Model file for the job. Use its own axes, mm. A direction names the side the tool comes from. Round coordinates to 2 decimals unless told otherwise and drop trailing zeros. Use one line per item in the form item = value.
from build123d import *

# Parameters (mm, degrees)
BOSS_EXTRU_1_DEPTH      = 2
CONG_1_R                = 10
ENL_V_MAT_EXTRU_1_DEPTH = 2
BOSS_EXTRU_2_DEPTH      = 0.6
CONG_2_R                = 10
ESQUISSE3_R             = 1.15
ENL_V_MAT_EXTRU_2_DEPTH = 10
CHANFREIN1_SIZE         = 0.5
CHANFREIN3_SIZE         = 0.6


with BuildPart() as part:
    # Esquisse1 → Boss.-Extru.1 (new body)
    with BuildSketch(Plane.XY):
        Polygon((-40.879571388, 34.615718895), (81.042798068, 34.615718895), (104.193503713, 7.025782272), (38.617977526, -93.674532757), (1.545249154, -93.674532757), (-64.030277033, 7.025782272), align=None)
    extrude(amount=BOSS_EXTRU_1_DEPTH)

    # Congé1
    cong_1_edges = [part.edges().sort_by_distance(p)[0] for p in [
        (-40.879571388, 34.615718895, 1),
        (81.042798068, 34.615718895, 1),
        (104.193503713, 7.025782272, 1),
        (38.617977526, -93.674532757, 1),
        (1.545249154, -93.674532757, 1),
        (-64.030277033, 7.025782272, 1),
    ]]
    fillet(cong_1_edges, radius=CONG_1_R)

    # Esquisse2 → Enlèv. mat.-Extru.1 (cut)
    with BuildSketch(Plane.XY.offset(2)):
        Polygon((-36.216494806, 24.615718895), (-51.607204261, 6.27378561), (6.96667711, -83.674532757), (33.19654957, -83.674532757), (91.770430941, 6.27378561), (76.379721487, 24.615718895), align=None)
    extrude(amount=-ENL_V_MAT_EXTRU_1_DEPTH, mode=Mode.SUBTRACT)

    # Esquisse4 → Boss.-Extru.2 (add)
    with BuildSketch(Plane(origin=(0, 0, 0), x_dir=(-1, 0, 0), z_dir=(0, 0, -1))):
        Polygon((-78.244952119, 28.615718895), (-96.73966005, 6.574584275), (-35.365120753, -87.674532757), (-4.798105928, -87.674532757), (56.57643337, 6.574584275), (38.081725439, 28.615718895), align=None)
        Polygon((-76.379721487, 24.615718895), (-91.770430941, 6.27378561), (-33.19654957, -83.674532757), (-6.96667711, -83.674532757), (51.607204261, 6.27378561), (36.216494806, 24.615718895), align=None, mode=Mode.SUBTRACT)
    extrude(amount=BOSS_EXTRU_2_DEPTH)

    # Congé2
    cong_2_edges = [part.edges().sort_by_distance(p)[0] for p in [
        (-36.216494806, 24.615718895, 0.7),
        (76.379721487, 24.615718895, 0.7),
        (91.770430941, 6.27378561, 0.7),
        (33.19654957, -83.674532757, 0.7),
        (6.96667711, -83.674532757, 0.7),
        (-51.607204261, 6.27378561, 0.7),
    ]]
    fillet(cong_2_edges, radius=CONG_2_R)

    # Esquisse3 → Enlèv. mat.-Extru.2 (cut)
    with BuildSketch(Plane.XY.offset(2)):
        with Locations((20.08161334, -91.058073416)):
            Circle(ESQUISSE3_R)
        with Locations((-28.872824595, -42.931783887)):
            Circle(ESQUISSE3_R)
        with Locations((20.08161334, 32.415718895)):
            Circle(ESQUISSE3_R)
        with Locations((90.076701777, 20.426939275)):
            Circle(ESQUISSE3_R)
        with Locations((69.036051275, -42.931783887)):
            Circle(ESQUISSE3_R)
        with Locations((-49.913475097, 20.426939275)):
            Circle(ESQUISSE3_R)
    extrude(amount=-ENL_V_MAT_EXTRU_2_DEPTH, mode=Mode.SUBTRACT)

    # Chanfrein1
    chanfrein1_edges = [part.edges().sort_by_distance(p)[0] for p in [
        (-51.063475097, 20.426939275, 2),
        (67.886051275, -42.931783887, 2),
        (88.926701777, 20.426939275, 2),
        (18.93161334, 32.415718895, 2),
        (-30.022824595, -42.931783887, 2),
        (18.93161334, -91.058073416, 2),
    ]]
    chamfer(chanfrein1_edges, length=CHANFREIN1_SIZE)

    # Chanfrein3
    chanfrein3_edges = [part.edges().sort_by_distance(p)[0] for p in [
        (87.492306084, 17.595151585, -0.6),
        (20.08161334, 28.615718895, -0.6),
        (-47.329079404, 17.595151585, -0.6),
        (-25.889163721, -40.549974241, -0.6),
        (20.08161334, -87.674532757, -0.6),
        (66.052390401, -40.549974241, -0.6),
    ]]
    chamfer(chanfrein3_edges, length=CHANFREIN3_SIZE - 0.0001)  # a hair under: the kernel refuses the full size


solid = part.part
(1) Pin check, flat tips, straight feed: pin 1 (1.5 mm diameter, centred on x = 78.5, z = 1.5, fed in from +Y); pin 2 (1.8 mm diameter, centred on x = 20.08, y = 32.42, fed in from +Z); pin 3 (3.5 mm diameter, centred on x = -28.87, y = -42.93, fed in from -Z); pin 4 (3 mm diameter, centred on x = 69.04, y = -42.93, fed in from +Z). Stop position of each tip, or through.
Report:
pin_1 = 34.52
pin_2 = through
pin_3 = 0
pin_4 = 1.85
(2) Slice it at B-B on z = 0.45. Count the separate pieces of the cut face and the enclosed holes in it, then the cut area to 3 significant figures.
Report:
separate_pieces = 1
enclosed_holes = 7
area = 4,340 mm2
(3) Pull direction Y, two halves, no side cores. Call faces 1 (the face through (7.56, -82.43, 0.72)), 2 (the face through (57, -48, 2)), 3 (the face through (80.55, 33.704, 1.014)), 4 (the face through (83.14, 16.56, 0.72)): released by +Y, released by -Y, zero draft, split by the parting line, or undercut.
Report:
face_1 = undercut
face_2 = zero draft
face_3 = released by +Y
face_4 = undercut
(4) Probe probe 1 along X at (y, z) = (20.5, 1.8); probe 2 along Y at (x, z) = (22, 1.45); probe 3 along Z at (x, y) = (75, -37.5). List the from-to ranges inside material, lowest first. Write a range as [from, to].
Report:
probe_1 = [-52.72, -51.36], [-48.47, -39.67], [79.83, 88.63], [91.52, 92.89]
probe_2 = [-93.67, -83.67], [24.62, 34.62]
probe_3 = [0, 2]
(5) Tool access for faces 5 (the face through (-21.417, -40.088, 0.718)), 6 (the face through (87.1, 17.6, -0.3)): list every direction of +Z, -Z, +X, -X, +Y, -Y with a clear straight run to the whole face (end or side of a thin tool).
Report:
face_5 = +Z, -Z
face_6 = -Z, +X, +Y
